For this review, take the finished solid that the model builds, in its own axes (mm). Face numbers are marked on the shaded views. A direction names the side the tool comes from. Give positions to 0.01 mm unless a question says otherwise; leave off trailing zeros. Write each loop counter-clockwise with the first axis right and the second up, starting at its lowest first coordinate (ties: lowest second). Pieces come first, ordered by that corner, then holes. Notation, with made-up numbers: M 28,-37.75 L 66,-37.75 A36 ccw 66,-1.75 Z; hole C -35,66 d2. An arc over 180 degrees is marked long. Write item = value, one per line.
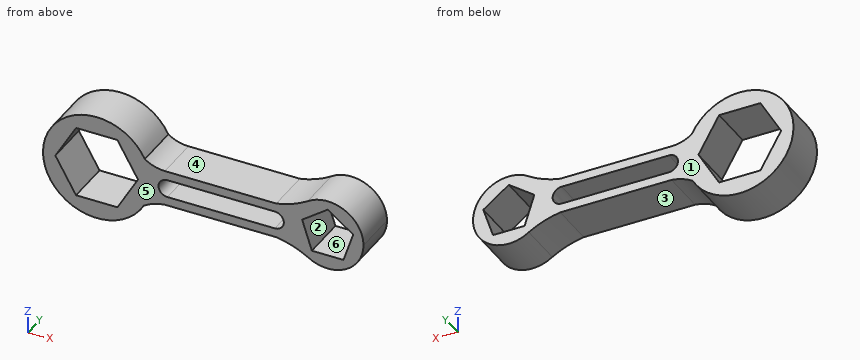
```python
from build123d import *

# Parameters (mm, degrees)
F1_DEPTH = 25


with BuildPart() as f1:
    # F0 (on Front) → F1 (new body)
    with BuildSketch(Plane.XZ):
        with BuildLine():
            ThreePointArc((-49.045524, -14.472526), (-46.269099, -7.471705), (-45.323765, 0))
            ThreePointArc((-45.323765, 0), (-46.116799, 6.852234), (-48.453973, 13.342198))
            ThreePointArc((-48.453973, 13.342198), (-105.316983, 0.637882), (-49.045524, -14.472526))
        make_face()
        Polygon((-98.417776, 0), (-86.870771, 20), (-63.77676, 20), (-52.229754, 0), (-63.77676, -20), (-86.870771, -20), align=None, mode=Mode.SUBTRACT)
        with BuildLine():
            ThreePointArc((-48.453973, 13.342198), (-46.116799, 6.852234), (-45.323765, 0))
            ThreePointArc((-45.323765, 0), (-46.269099, -7.471705), (-49.045524, -14.472526))
            ThreePointArc((-49.045524, -14.472526), (-43.387683, -11.643077), (-37.214165, -10.262998))
            Line((-37.214165, -10.262998), (24.944222, -10.262998))
            ThreePointArc((24.944222, -10.262998), (34.03408, -12.573077), (42.50839, -16.591542))
            ThreePointArc((42.50839, -16.591542), (33.676235, 0), (42.50839, 16.591542))
            ThreePointArc((42.50839, 16.591542), (34.063025, 12.301459), (24.944222, 9.737002))
            Line((24.944222, 9.737002), (-37.214165, 9.737002))
            ThreePointArc((-37.214165, 9.737002), (-43.116087, 10.660362), (-48.453973, 13.342198))
        make_face()
        with BuildLine():
            ThreePointArc((-40.823765, -0.262998), (-39.359299, 3.272535), (-35.823765, 4.737002))
            Line((-35.823765, 4.737002), (24.176235, 4.737002))
            ThreePointArc((24.176235, 4.737002), (27.711769, 3.272535), (29.176235, -0.262998))
            ThreePointArc((29.176235, -0.262998), (27.711769, -3.798532), (24.176235, -5.262998))
            Line((24.176235, -5.262998), (-35.823765, -5.262998))
            ThreePointArc((-35.823765, -5.262998), (-39.359299, -3.798532), (-40.823765, -0.262998))
        make_face(mode=Mode.SUBTRACT)
        with BuildLine():
            ThreePointArc((73.676235, 0), (63.07419, 17.654417), (42.50839, 16.591542))
            ThreePointArc((42.50839, 16.591542), (33.676235, 0), (42.50839, -16.591542))
            ThreePointArc((42.50839, -16.591542), (63.07419, -17.654417), (73.676235, 0))
        make_face()
        Polygon((53.676235, 15), (67.942083, 4.635255), (62.493014, -12.135255), (44.859456, -12.135255), (39.410387, 4.635255), align=None, mode=Mode.SUBTRACT)
    extrude(amount=F1_DEPTH)


solid = f1.part
```
1. We need section B-B, the plane y = -13.5. Write out the cut boundary in (x, z), then the cut area to 3 significant figures.
Responses:
outline = M -49.05,-14.47 A26.01 cw -37.21,-10.26 L 24.94,-10.26 A48.44 cw 42.51,-16.59 A20 ccw long 42.51,16.59 A48.44 cw 24.94,9.74 L -37.21,9.74 A19.32 cw -48.45,13.34 A30 ccw long Z; hole M -98.42,0 L -86.87,-20 L -63.78,-20 L -52.23,0 L -63.78,20 L -86.87,20 Z; hole M -40.82,-0.26 A5 ccw -35.82,-5.26 L 24.18,-5.26 A5 ccw 29.18,-0.26 A5 ccw 24.18,4.74 L -35.82,4.74 A5 ccw Z; hole M 39.41,4.64 L 44.86,-12.14 L 62.49,-12.14 L 67.94,4.64 L 53.68,15 Z
area = 3,160 mm2
2. Machinability: for the marked faces 3, 4, 5 and 6, which of the approach directions +Z, -Z, +X, -X, +Y, -Y give a long, thin tool a straight path to every point of the face, cutting with its end or side? Answer none if there is none.
Responses:
face_3 = -Z, +Y, -Y
face_4 = +Z, +Y, -Y
face_5 = +Z, -Z, +X, -X, -Y
face_6 = +Y, -Y
3. The part is to be moulded in two halves that separate along X. For the marked faces 1 and 2, say which applies: +X half, -X half, draft (parallel to the pull), parting line (faces both ways), or undercut.
Responses:
face_1 = draft
face_2 = undercut
4. We need section A-A, the plane x = 6. Write out the cut boundary in (y, z).
Responses:
outline = M -25,-10.26 L 0,-10.26 L 0,-5.26 L -25,-5.26 Z; M -25,4.74 L 0,4.74 L 0,9.74 L -25,9.74 Z
5. For line 1 along Z through (x, y) = (-6, -7); line 2 along X through (y, z) = (-5, 4); line 3 along X through (y, z) = (-18, -8), list the stretches that pass through material, from the lowest coordinate up. Write a range as from..to.
Responses:
line_1 = -10.26..-5.26, 4.74..9.74
line_2 = -105.06..-96.11, -54.54..-38.44, 26.79..39.62, 67.74..73.27
line_3 = -104.24..-93.8, -56.85..43.52, 63.84..72.01
6. Insertion check: P1, Ø6, axis at x = 44.5, z = -14.5, coming from the +Y side; P2, Ø7.5, axis at x = 8, y = -10.5, coming from the -Z side; P3, Ø3, axis at y = -6, z = 17.5, coming from the -X side; P4, Ø12.5, axis at x = -12.5, y = -17, coming from the +Z side. Each pin has a flat end and moves straight along its axis. Give the tip position at first contact, or say it passes through.
Responses:
P1 = 0
P2 = -10.26
P3 = -100.7
P4 = 9.74
7. We need section D-D, the plane x = 47. Write out the cut boundary in (y, z), then the cut area to 3 significant figures.
Responses:
outline = M -25,-18.85 L 0,-18.85 L 0,-12.14 L -25,-12.14 Z; M -25,10.15 L 0,10.15 L 0,18.85 L -25,18.85 Z
area = 386 mm2
8. We need section C-C, the plane z = -2.5. Write out the cut boundary in (x, y), then the cut area to 3 significant figures.
Responses:
outline = M -105.22,-25 L -96.97,-25 L -96.97,0 L -105.22,0 Z; M -53.67,-25 L -40.3,-25 L -40.3,0 L -53.67,0 Z; M 28.65,-25 L 41.73,-25 L 41.73,0 L 28.65,0 Z; M 65.62,-25 L 73.52,-25 L 73.52,0 L 65.62,0 Z
area = 1,060 mm2
